from build123d import *

# Parameters (mm, degrees)
BOSS_EXTRUDE1_DEPTH = 2.54
BOSS_EXTRUDE3_DEPTH = 2.794
BOSS_EXTRUDE4_DEPTH = 2.794
CUT_EXTRUDE1_DEPTH  = 2.794
CUT_EXTRUDE2_DEPTH  = 2.794
CUT_EXTRUDE3_DEPTH  = 2.794
CUT_EXTRUDE4_DEPTH  = 2.794


with BuildPart() as part:
    # Sketch2 → Boss-Extrude1 (new body)
    with BuildSketch(Plane(origin=(0, 0, 0), x_dir=(1, 0, 0), z_dir=(0, 1, 0))):
        Polygon((-1.905, 0), (1.905, 0), (1.905, 24.289959425), (2.748388443, 25.169443727), (18.139363721, 33.964286743), (20.066, 37.152417336), (20.066, 90.357876746), (16.27045958, 90.357876746), (16.27045958, 37.152417336), (0, 27.917832169), (-16.380395118, 37.152417336), (-16.380395118, 90.357876746), (-20.066, 90.357876746), (-20.066, 37.152417336), (-18.359234796, 33.964286743), (-2.748388443, 25.169443727), (-1.905, 24.289959425), align=None)
    extrude(amount=BOSS_EXTRUDE1_DEPTH)

    # Sketch3 → Boss-Extrude3 (add)
    with BuildSketch(Plane(origin=(0, 2.54, 0), x_dir=(1, 0, 0), z_dir=(0, 1, 0))):
        Polygon((-20.066, 64.416430686), (-23.843651965, 64.416430686), (-24.093769894, 64.416430686), (-24.093769894, 34.012983608), (-18.385304655, 34.012983608), (-20.066, 37.152417336), align=None)
    extrude(amount=-BOSS_EXTRUDE3_DEPTH)

    # Sketch5 → Boss-Extrude4 (add)
    with BuildSketch(Plane(origin=(0, 2.54, 0), x_dir=(1, 0, 0), z_dir=(0, 1, 0))):
        Polygon((23.79791373, 64.416430686), (20.066, 64.416430686), (20.066, 37.152417336), (18.139363721, 33.964286743), (17.94697653, 33.854351205), (23.79791373, 33.854351205), align=None)
    extrude(amount=-BOSS_EXTRUDE4_DEPTH)

    # Sketch6 → Cut-Extrude1 (cut)
    with BuildSketch(Plane(origin=(0, 2.54, 0), x_dir=(1, 0, 0), z_dir=(0, 1, 0))):
        Polygon((-16.380395118, 37.152417336), (-19.425262821, 39.079248043), (-19.425262821, 61.216281017), (-16.380395118, 63.274089716), align=None)
    extrude(amount=-CUT_EXTRUDE1_DEPTH, mode=Mode.SUBTRACT)

    # Sketch7 → Cut-Extrude2 (cut)
    with BuildSketch(Plane(origin=(0, 2.54, 0), x_dir=(1, 0, 0), z_dir=(0, 1, 0))):
        Polygon((16.27045958, 37.152417336), (19.210779399, 39.131257015), (19.210779399, 60.348815791), (16.022648806, 63.536946385), align=None)
    extrude(amount=-CUT_EXTRUDE2_DEPTH, mode=Mode.SUBTRACT)

    # Sketch8 → Cut-Extrude3 (cut)
    with BuildSketch(Plane(origin=(0, 2.54, 0), x_dir=(1, 0, 0), z_dir=(0, 1, 0))):
        Polygon((-18.359234796, 33.964286743), (-25.982779442, 39.241192553), (-25.982779442, 59.799138103), (-20.066, 64.416430686), (-26.704115548, 65.235310973), (-32.139169553, 50.784424011), (-24.093769894, 30.886091687), align=None)
    extrude(amount=-CUT_EXTRUDE3_DEPTH, mode=Mode.SUBTRACT)

    # Sketch9 → Cut-Extrude4 (cut)
    with BuildSketch(Plane(origin=(0, 2.54, 0), x_dir=(1, 0, 0), z_dir=(0, 1, 0))):
        Polygon((17.94697653, 33.854351205), (23.79791373, 37.9219661), (26.535723591, 53.149224599), (25.166818661, 60.568686867), (20.066, 64.416430686), (22.61640933, 67.797418641), (32.063184465, 64.416430686), (29.094924947, 33.854351205), (20.441248246, 27.838251042), align=None)
    extrude(amount=-CUT_EXTRUDE4_DEPTH, mode=Mode.SUBTRACT)


solid = part.part
Source: CAD feature listing. Evaluate the final solid. Frame: model axes, mm. A direction names the side the tool comes from. Give positions to 0.01 mm unless a question says otherwise; leave off trailing zeros. Write each loop counter-clockwise with the first axis right and the second up, starting at its lowest first coordinate (ties: lowest second). Pieces come first, ordered by that corner, then holes. Notation, with made-up numbers: M 54.5,57 L 108.5,57 A27 cw 108.5,90 Z; hole C -22,17 d4. An arc over 180 degrees is marked long. Return JSON: item names as keys, results as strings. Group by question number.
1) Cut plane D-D, the plane x = 6. Output: boundary loops of the cut face in (y, z).
2) Set-up query: faces 1 (the face through (23.798, 1, -50)), 2 (the face through (19.211, 1, -50)), 3 (the face through (-1.905, 1, -12)), 4 (the face through (16.27, 1, -77)). Return all of +Z, -Z, +X, -X, +Y, -Y with unobstructed straight access to the full face (end or side cutting, diameter ignored); none if empty.
3) Material intervals for line 1 along X through (y, z) = (1.9, -47.5); line 2 along X through (y, z) = (0.1, -71.5); line 3 along X through (y, z) = (1.15, -23.5) (3 decimals), sorted ascending. Write a range as [from, to].
4) Cut plane A-A, the plane z = -56. Output: boundary loops of the cut face in (x, y), plus the area to 3 significant figures.
5) Pull-direction query (X, two-part tool) for faces 5 (the face through (8.25, 1.25, -32.6)), 6 (the face through (-18, 1, -90.358)), 7 (the face through (1.905, 1, -12)); classes: pulls with the +X half, pulls with the -X half, needs draft (parallel to the pull), parting line crosses it, or undercut.
6) Cut plane C-C, the plane z = -75. Output: boundary loops of the cut face in (x, y).
7) Pin query (flat end, axial travel): P1, Ø1, axis at y = 0, z = -76, coming from the +X side; P2, Ø1, axis at x = -6.5, y = 1.5, coming from the +Z side; P3, Ø0.8, axis at y = 1.5, z = -18, coming from the +X side (3 decimals); P4, Ø1, axis at x = 14.5, z = -79.5, coming from the +Y side. Return the tip coordinate at first contact, or that it passes through.
Recorded:
{
 "1": {"outline": "M 0,-31.32 L 2.54,-31.32 L 2.54,-27.03 L 0,-27.03 Z"},
 "2": {"face 1": "+Z, -Z, +X, +Y, -Y", "face 2": "+Y, -Y", "face 3": "+Z, -X, +Y, -Y", "face 4": "-Z, +Y, -Y"},
 "3": {"line 1": "x = [-24.09, -19.43], [19.21, 23.8]", "line 2": "x = [-20.07, -16.38], [16.27, 20.07]", "line 3": "x = [-1.905, 1.905]"},
 "4": {"outline": "M -24.09,-0.25 L -20.07,-0.25 L -20.07,0 L -19.43,0 L -19.43,2.54 L -24.09,2.54 Z; M 19.21,0 L 20.07,0 L 20.07,-0.25 L 23.8,-0.25 L 23.8,2.54 L 19.21,2.54 Z", "area": "25.5 mm²"},
 "5": {"face 5": "undercut", "face 6": "needs draft", "face 7": "pulls with the +X half"},
 "6": {"outline": "M -20.07,0 L -16.38,0 L -16.38,2.54 L -20.07,2.54 Z; M 16.27,0 L 20.07,0 L 20.07,2.54 L 16.27,2.54 Z"},
 "7": {"P1": "stops at x = 20.07", "P2": "stops at z = -27", "P3": "stops at x = 1.905", "P4": "passes through"}
}
